```python
from build123d import *

# Parameters (mm, degrees)
CUT_EXTRUDE_1_DEPTH = 2.5


with BuildPart() as part:
    # 草图2 → 旋转1 (revolve)
    with BuildSketch(Plane(origin=(0, 0, 0), x_dir=(0, 0, -1), z_dir=(1, 0, 0)), mode=Mode.PRIVATE) as revolve_1_sk:
        Polygon((6, 9.5), (0, 9.5), (0, 0), (30, 0), (30, 6), (6, 6), align=None)
    revolve(revolve_1_sk.sketch.rotate(Axis((0, 0, 0), (0, 0, -1)), 90), axis=Axis((0, 0, 0), (0, 0, -1)))

    # 草图3 → 切除-拉伸1 (cut)
    with BuildSketch(Plane.XY):
        Polygon((2.193931023, -3.8), (4.387862046, 0), (2.193931023, 3.8), (-2.193931023, 3.8), (-4.387862046, 0), (-2.193931023, -3.8), align=None)
    extrude(amount=-CUT_EXTRUDE_1_DEPTH, mode=Mode.SUBTRACT)

    # 草图4 → 切除-旋转1 (revolve, cut)
    with BuildSketch(Plane(origin=(0, 0, 0), x_dir=(0, 0, -1), z_dir=(1, 0, 0)), mode=Mode.PRIVATE) as cut_revolve_1_sk:
        with BuildLine():
            Line((6, 9.5), (0, 9.5))
            Line((0, 9.5), (0, 6))
            ThreePointArc((0, 6), (2.526889003, 8.561047424), (6, 9.5))
        make_face()
    revolve(cut_revolve_1_sk.sketch.rotate(Axis((0, 0, 0), (0, 0, -1)), 90), axis=Axis((0, 0, 0), (0, 0, -1)), mode=Mode.SUBTRACT)


solid = part.part
```
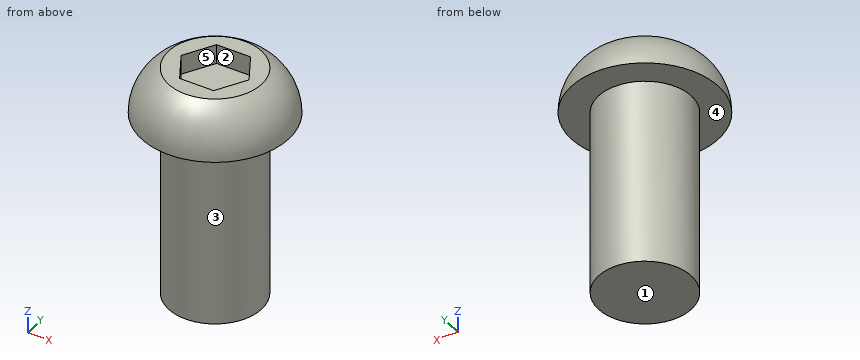
For this review, take the finished solid that the model builds, in its own axes (mm). Face numbers are marked on the shaded views. A direction names the side the tool comes from. Round coordinates to 2 decimals unless told otherwise and drop trailing zeros. Write each loop counter-clockwise with the first axis right and the second up, starting at its lowest first coordinate (ties: lowest second). Pieces come first, ordered by that corner, then holes.
1) Mouldability with a two-part tool opening along Y and no side actions: class the marked faces 3, 4 and 5 as +Y half, -Y half, draft (parallel to the pull), parting line (faces both ways), or undercut.
Answer below:
face 3: parting line
face 4: draft
face 5: undercut
2) Machinability: for the marked faces 1 and 2, which of the approach directions +Z, -Z, +X, -X, +Y, -Y give a long, thin tool a straight path to every point of the face, cutting with its end or side? Answer none if there is none.
Answer below:
face 1: -Z, +X, -X, +Y, -Y
face 2: +Z
3) Insertion check: pin 1 Ø1.5 at (x, z) = (6, -14.5) entering from +Y; pin 2 Ø6 at (x, y) = (-0.5, -0.5) entering from +Z; pin 3 Ø5 at (x, z) = (6, -18) entering from +Y. Each pin has a flat end and moves straight along its axis. Give the tip position at first contact, or say it passes through.
Answer below:
pin 1: stops at y = 2.9
pin 2: stops at z = -2.5
pin 3: stops at y = 4.87
4) For line 1 along Y through (x, z) = (0.25, -25.5); line 2 along X through (y, z) = (3.5, -25.5); line 3 along X through (y, z) = (7.5, -4), list the stretches that pass through material, from the lowest coordinate up.
Answer below:
line 1: y = -5.99 to 5.99
line 2: x = -4.87 to 4.87
line 3: x = -5.33 to 5.33
5) Take a section at A-A on z = -12. Give the boundary of the cut face in (x, y), then the cut area to 3 significant figures.
Answer below:
outline: circle Ø12 at (0, 0)
area: 113 mm2
